```python
from build123d import *

# Parameters (mm, degrees)
F1_DEPTH = 6.35
F0_R     = 11.049
F2_DEPTH = 6.35
F3_DEPTH = 6.35
F4_DEPTH = 6.35
F5_DEPTH = 6.35


with BuildPart() as f1:
    # F0 (on Top) → F1 (new body)
    with BuildSketch(Plane.XY):
        with BuildLine():
            ThreePointArc((11.760597, 21.670156), (6.701838, 16.952502), (0, 15.24))
            ThreePointArc((0, 15.24), (-6.836853, 17.027293), (-11.924319, 21.931847))
            ThreePointArc((-11.924319, 21.931847), (-12.914458, 8.219461), (-23.310372, -0.77692))
            ThreePointArc((-23.310372, -0.77692), (-14.739412, -5.455867), (-11.326602, -14.605))
            ThreePointArc((-11.326602, -14.605), (-11.734078, -17.954455), (-12.932736, -21.108517))
            ThreePointArc((-12.932736, -21.108517), (0.641019, -15.443026), (13.646185, -22.313999))
            ThreePointArc((13.646185, -22.313999), (13.101766, -7.789805), (25.757442, -0.642603))
            ThreePointArc((25.757442, -0.642603), (13.520656, 7.227739), (11.760597, 21.670156))
        make_face()
        with BuildLine():
            ThreePointArc((13.97, 0), (-9.878282, -9.878282), (0, 13.97))
            ThreePointArc((0, 13.97), (9.878282, 9.878282), (13.97, 0))
        make_face(mode=Mode.SUBTRACT)
    extrude(amount=F1_DEPTH)

    # F0 (on Top) → F2 (join)
    with BuildSketch(Plane.XY):
        with BuildLine():
            ThreePointArc((-11.326602, -14.605), (-14.739412, -5.455867), (-23.310372, -0.77692))
            ThreePointArc((-23.310372, -0.77692), (-38.496664, -19.178757), (-15.180625, -24.239724))
            ThreePointArc((-15.180625, -24.239724), (-14.144468, -22.611098), (-12.932736, -21.108517))
            ThreePointArc((-12.932736, -21.108517), (-11.734078, -17.954455), (-11.326602, -14.605))
        make_face()
        with Locations((-25.296602, -14.605)):
            Circle(F0_R, mode=Mode.SUBTRACT)
    extrude(amount=F2_DEPTH)

    # F0 (on Top) → F3 (join)
    with BuildSketch(Plane.XY):
        with BuildLine():
            ThreePointArc((27.282832, -0.77692), (26.518634, -0.726829), (25.757442, -0.642603))
            ThreePointArc((25.757442, -0.642603), (13.101766, -7.789805), (13.646185, -22.313999))
            ThreePointArc((13.646185, -22.313999), (29.321808, -27.982541), (39.266602, -14.605))
            ThreePointArc((39.266602, -14.605), (35.853792, -5.455867), (27.282832, -0.77692))
        make_face()
        with Locations((25.296602, -14.605)):
            Circle(F0_R, mode=Mode.SUBTRACT)
    extrude(amount=F3_DEPTH)

    # F0 (on Top) → F4 (join)
    with BuildSketch(Plane.XY):
        with BuildLine():
            ThreePointArc((-11.924319, 21.931847), (-6.836853, 17.027293), (0, 15.24))
            ThreePointArc((0, 15.24), (6.701838, 16.952502), (11.760597, 21.670156))
            ThreePointArc((11.760597, 21.670156), (12.469752, 23.474968), (13.378501, 25.187983))
            ThreePointArc((13.378501, 25.187983), (13.821334, 27.177361), (13.97, 29.21))
            ThreePointArc((13.97, 29.21), (-2.032639, 43.031334), (-13.378501, 25.187983))
            ThreePointArc((-13.378501, 25.187983), (-12.57041, 23.59609), (-11.924319, 21.931847))
        make_face()
        with BuildLine():
            ThreePointArc((11.049, 29.21), (7.812823, 21.397177), (0, 18.161))
            ThreePointArc((0, 18.161), (-7.812823, 37.022823), (11.049, 29.21))
        make_face(mode=Mode.SUBTRACT)
    extrude(amount=F4_DEPTH)

    # F0 (on Top) → F5 (join)
    with BuildSketch(Plane.XY):
        with BuildLine():
            ThreePointArc((13.97, 0), (9.878282, 9.878282), (0, 13.97))
            ThreePointArc((0, 13.97), (-9.878282, -9.878282), (13.97, 0))
        make_face()
        with BuildLine():
            ThreePointArc((0, 11.049), (7.812823, 7.812823), (11.049, 0))
            ThreePointArc((11.049, 0), (-7.812823, -7.812823), (0, 11.049))
        make_face(mode=Mode.SUBTRACT)
    extrude(amount=F5_DEPTH)


solid = f1.part
```
The model under review builds one solid part; all positions refer to its coordinate system, in mm. A direction names the side the tool comes from. Give positions to 0.01 mm unless a question says otherwise; leave off trailing zeros. Loops run counter-clockwise (first coordinate to the right, second up) from the corner with the lowest first, then second, coordinate; pieces in that order, holes last. Notation, with made-up numbers: (68, -10) -> (89, -10) arc R30 ccw to (89, 29) -> close; hole circle Ø1 at (44, 5.25). An arc over 180 degrees is marked (long way). Use CSV: the item, a comma, the result in double quotes.
1. To check wall thickness, follow probe 1 along Y at (x, z) = (0, 4); probe 2 along X at (y, z) = (29.5, 2.5); probe 3 along Y at (x, z) = (-4, 2.75). State the ranges of each line that lie inside material, in increasing order. Write a range as from..to.
Result:
probe 1,"y = -15.43..-11.05, 11.05..18.16, 40.26..43.18"
probe 2,"x = -13.97..-11.05, 11.05..13.97"
probe 3,"y = -15.86..-10.3, 10.3..18.91, 39.51..42.6"
2. Consider section B-B, the plane y = 8.5. Write out the cut boundary in (x, z), then the cut area to 3 significant figures.
Result:
outline,"(-12.78, 0) -> (-7.06, 0) -> (-7.06, 6.35) -> (-12.78, 6.35) -> close; (7.06, 0) -> (12.8, 0) -> (12.8, 6.35) -> (7.06, 6.35) -> close"
area,"72.7 mm²"
3. Consider section D-D, the plane x = -21. Write out the cut boundary in (y, z).
Result:
outline,"(-27.9, 0) -> (-24.78, 0) -> (-24.78, 6.35) -> (-27.9, 6.35) -> close; (-4.43, 0) -> (0.17, 0) -> (0.17, 6.35) -> (-4.43, 6.35) -> close"
4. The part is to be moulded in two halves that separate along Y. For faces 1 (the face through (9, 7, 0)), 2 (the face through (-12.58, 23.62, 3.13)), 3 (the face through (-38.62, -18.8, 3.13)), 4 (the face through (13.817, 27.149, 3.131)), say which applies: +Y half, -Y half, draft (parallel to the pull), parting line (faces both ways), or undercut.
Result:
face 1,"draft"
face 2,"undercut"
face 3,"parting line"
face 4,"undercut"
5. Consider section C-C, the plane z = 1.75. Write out the cut boundary in (x, y) (1 decimal), then the cut area to 3 significant figures.
Result:
outline,"(-23.3, -0.8) arc R14 ccw (long way) to (-15.2, -24.2) arc R17.2 cw to (-12.9, -21.1) arc R17.2 cw to (13.6, -22.3) arc R14 ccw to (39.3, -14.6) arc R14 ccw to (27.3, -0.8) arc R17.1 cw to (25.8, -0.6) arc R17.1 cw to (11.8, 21.7) arc R17.1 cw to (13.4, 25.2) arc R14 ccw to (14, 29.2) arc R14 ccw (long way) to (-13.4, 25.2) arc R18 cw to (-11.9, 21.9) arc R18 cw to start; hole circle Ø22.1 at (-25.3, -14.6); hole circle Ø22.1 at (0, 0); hole circle Ø22.1 at (0, 29.2); hole circle Ø22.1 at (25.3, -14.6)"
area,"1,260 mm²"
6. For P1, Ø2, axis at x = -29, z = 5.5, coming from the -Y side; P2, Ø1.5, axis at x = 24, z = 2.5, coming from the +Y side; P3, Ø3, axis at x = 27, z = 3.5, coming from the -Y side; P4, Ø10, axis at x = 17, y = 29.5, coming from the +Z side, all flat-tipped, find the tip position at first contact; note any pin that passes through.
Result:
P1,"stops at y = -28.31"
P2,"stops at y = -0.11"
P3,"stops at y = -28.57"
P4,"stops at z = 6.35"
7. Machinability: for faces 5 (the face through (-33.44, -7.14, 3.13)), 6 (the face through (12.46, 23.45, 3.13)), which of the approach directions +Z, -Z, +X, -X, +Y, -Y give a long, thin tool a straight path to every point of the face, cutting with its end or side? Answer none if there is none.
Result:
face 5,"+Z, -Z"
face 6,"+Z, -Z, +X"
8. Consider section A-A, the plane x = -8. Write out the cut boundary in (y, z).
Result:
outline,"(-17.32, 0) -> (-7.62, 0) -> (-7.62, 6.35) -> (-17.32, 6.35) -> close; (7.62, 0) -> (21.59, 0) -> (21.59, 6.35) -> (7.62, 6.35) -> close; (36.83, 0) -> (40.66, 0) -> (40.66, 6.35) -> (36.83, 6.35) -> close"
